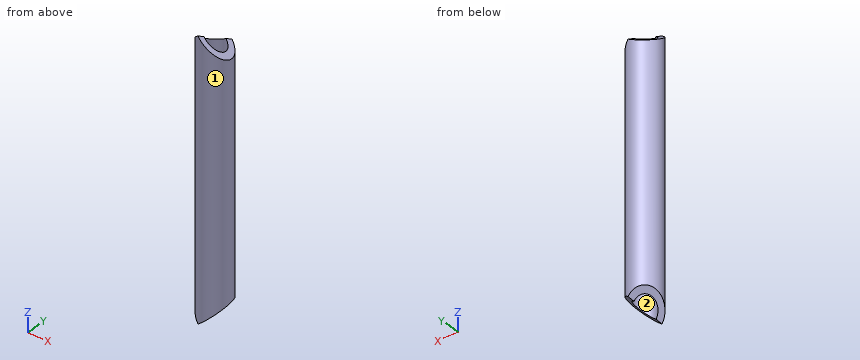
Autodesk Inventor part; units mm, degrees
ref_plane "Start Plane" through (0, 0, -4.9897) normal (0, 0, 1) x (1, 0, 0)
ref_plane "End Plane" through (0, 0, 183.044) normal (0, 0, 1) x (1, 0, 0)
ref_plane "Work Plane4" through (-10.464, -2.0762, 187.8032) normal (0.6617, 0.1313, 0.7382) x (0.7481, -0.05, -0.6617)
ref_plane "Start Plane" through (0, 0, -4.9897) normal (0, 0, 1) x (1, 0, 0)
ref_plane "End Plane" through (0, 0, 183.044) normal (0, 0, 1) x (1, 0, 0)
sketch "Sketch" plane through (0, 0, 0) normal (0, 0, 1) x (1, 0, 0)
  circle A0 centre (0, 0) radius 6.9342
  circle A1 centre (0, 0) radius 10.668
  dimension "d0" = 21.336
  dimension "d1" = 3.7338
extrude "Body" add sketch "Sketch" along normal up to surface (188.0337 mm away) from surface at -4.9897
sketch "Sketch3" plane through (0, 0, 0) normal (0, 0, 1) x (1, 0, 0)
  line L0 (0, 0) -> (10, 0)
ref_plane "Work Plane3" through (0, 0, 0) normal (0, -1, 0) x (1, 0, 0)
sketch "Sketch4" plane through (0, 0, 0) normal (0, -1, 0) x (1, 0, 0)
  line L0 (-2, -4.9897) -> (12, -4.9897)
  line L1 (-2, 183.044) -> (12, 183.044)
  dimension "d7" = 188.0337
ref_plane "Work Plane4" through (-10.464, -2.0762, 187.8032) normal (0.6617, 0.1313, 0.7382) x (0.7481, -0.05, -0.6617)
split "Split1" plane through (-10.464, -2.0762, 187.8032) removes the side toward (0.6617, 0.1313, 0.7382)
ref_plane "Work Plane5" through (6.4449, -8.5011, 187.1496) normal (-0.392, 0.517, 0.761) x (0.9128, 0.1151, 0.392)
split "Split2" plane through (6.4449, -8.5011, 187.1496) removes the side toward (-0.392, 0.517, 0.761)
ref_plane "Work Plane6" through (-10.464, -2.0762, -9.7489) normal (0.6617, 0.1313, -0.7382) x (-0.6724, -0.3318, -0.6617)
split "Split3" plane through (-10.464, -2.0762, -9.7489) removes the side toward (0.6617, 0.1313, -0.7382)
ref_plane "Work Plane7" through (6.4449, -8.5011, -9.0952) normal (-0.392, 0.517, -0.761) x (0.3573, 0.8478, 0.392)
split "Split4" plane through (6.4449, -8.5011, -9.0952) removes the side toward (-0.392, 0.517, -0.761)
equation "\"d0\" = G_H"
equation "\"d1\" = G_T"
equation "\"d2\" = G_L"
equation "\"G_H\" = 21.336"
equation "\"G_T\" = 3.7338"
equation "\"G_L\" = 188.03367"
equation "\"G_OFFSET_START\" = 4.98966"
equation "\"G_OFFSET_END\" = 4.98966"
equation "\"d4\" = -G_OFFSET_START"
equation "\"d5\" = G_OFFSET_END + B_L"
equation "\"B_L\" = 178.05435"
properties part number "ANSI - 1/2 x 0.147 - 7.403" material "Steel, Mild"
Geometry check sheet. Reference: the model listing, model coordinates, mm. Face numbers are marked on the shaded views. Coordinates: 2 decimals unless noted, no trailing zeros. Order: outer loops, then holes, each group sorted by start corner. A loop starts at its lowest first (then second) coordinate and runs counter-clockwise, first axis right, second up. Notation, with made-up numbers: (1, -22) -> (9, -22) arc R15 cw to (9, 4) -> close; hole circle Ø5 at (86.5, 68.25). An arc over 180 degrees is marked (long way). Use a Markdown table: item, result. Add a question column.
1. Cross-section at A-A (y = 0). Enter the section's corners in (x, z), and give its area (3 significant figures).
2. Cross-section at B-B (x = 0). Enter the section's corners in (y, z).
3. Cross-section at C-C (z = 21.5). Enter the section's corners in (x, y).
4. Mould release check, pull along Y, two halves, no side actions. Record for the marked faces 1 and 2: pulls with the +Y half, pulls with the -Y half, needs draft (parallel to the pull), parting line crosses it, or undercut.
5. Material ranges on L1, parallel to X at y = 0, z = 84; L2, parallel to X at y = -1.75, z = 11.5, recorded low to high.
6. Go/stop test with flat-tipped pins: pin 1 Ø4 at (x, z) = (7, 135.5) entering from +Y; pin 2 Ø3 at (x, z) = (5.5, 107.5) entering from +Y; pin 3 Ø4 at (x, z) = (2.5, 110) entering from -Y. Record where each tip stops, or that it passes through.
Filled sheet:
| question | item | result |
|---|---|---|
| 1 | outline | (-10.67, 5.5) -> (-6.93, 3.57) -> (-6.93, 174.48) -> (-10.67, 172.56) -> close; (6.93, 6.22) -> (10.67, 9.56) -> (10.67, 168.49) -> (6.93, 171.84) -> close |
| 1 | area | 1,240 mm2 |
| 2 | outline | (-10.67, -1.9) -> (-6.93, -1.23) -> (-6.93, 179.29) -> (-10.67, 179.95) -> close; (6.93, 4.71) -> (10.67, 7.25) -> (10.67, 170.81) -> (6.93, 173.34) -> close |
| 3 | outline | circle Ø21.34 at (0, 0); hole circle Ø13.87 at (0, 0) |
| 4 | face 1 | parting line crosses it |
| 4 | face 2 | undercut |
| 5 | L1 | -10.67 to -6.93, 6.93 to 10.67 |
| 5 | L2 | -10.52 to -6.71, 6.71 to 10.52 |
| 6 | pin 1 | y = 9.42 |
| 6 | pin 2 | y = 9.89 |
| 6 | pin 3 | y = -10.66 |
